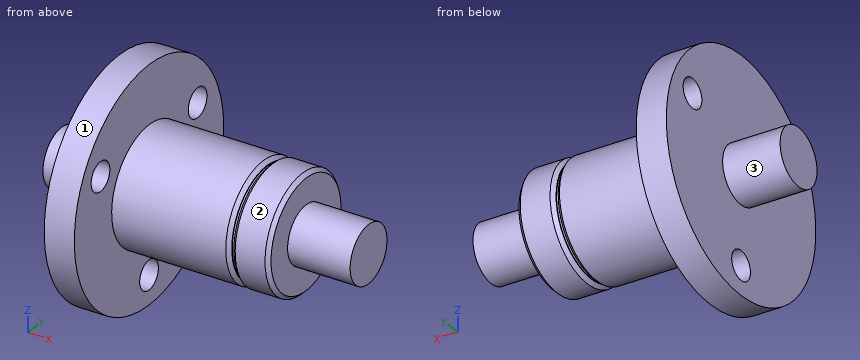
from build123d import *

# Parameters (mm, degrees)
SKETCH1_W          = 6.3
SKETCH1_H          = 3.133597909
SKETCH1_W_2        = 20.5
SKETCH1_W_3        = 6.85
SKETCH2_R          = 1.59
CUT_EXTRUDE1_DEPTH = 10
CIRPATTERN1_COUNT  = 3
CHAMFER1_SIZE      = 0.4


with BuildPart() as part:
    # Sketch1 → Revolve1 (revolve)
    with BuildSketch(Plane.XY, mode=Mode.PRIVATE) as revolve1_sk:
        with Locations((-6.45, 1.566798955)):
            Rectangle(SKETCH1_W, SKETCH1_H)
        with Locations((6.95, 1.566798955)):
            Rectangle(SKETCH1_W_2, SKETCH1_H)
        Polygon((17.2, 3.133597909), (17.2, 6.35), (13.132231879, 6.35), (13.132231879, 5.859469346), (12.9, 5.859469346), (12.9, 6.35), (0, 6.35), (0, 12.7), (-3.3, 12.7), (-3.3, 3.133597909), align=None)
        with Locations((20.625, 1.566798955)):
            Rectangle(SKETCH1_W_3, SKETCH1_H)
    revolve(revolve1_sk.sketch.rotate(Axis((-3.3, 0, 0), (1, 0, 0)), 90), axis=Axis((-3.3, 0, 0), (1, 0, 0)))

    # Sketch2 → Cut-Extrude1 (cut)
    with BuildSketch(Plane(origin=(0, 0, 0), x_dir=(0, 0, -1), z_dir=(1, 0, 0))):
        with Locations((9.525, 0)):
            Circle(SKETCH2_R)
    cut_extrude1 = extrude(amount=-CUT_EXTRUDE1_DEPTH, mode=Mode.SUBTRACT)

    # CirPattern1: Cut-Extrude1 ×3 about axis
    cirpattern1_axis = Axis((0, 0, 0), (1, 0, 0))
    for i in range(1, CIRPATTERN1_COUNT):
        add(cut_extrude1.rotate(cirpattern1_axis, i * 360 / CIRPATTERN1_COUNT), mode=Mode.SUBTRACT)

    # Chamfer1
    chamfer1_edges = [part.edges().sort_by_distance(p)[0] for p in [
        (12.9, 0, -6.35),
        (13.132231879, 0, -6.35),
        (17.2, 0, -6.35),
    ]]
    chamfer(chamfer1_edges, length=CHAMFER1_SIZE)


solid = part.part
The model under review builds one solid part; all positions refer to its coordinate system, in mm. Face numbers are marked on the shaded views. A direction names the side the tool comes from. Give positions to 0.01 mm unless a question says otherwise; leave off trailing zeros. Order: outer loops, then holes, each group sorted by start corner. A loop starts at its lowest first (then second) coordinate and runs counter-clockwise, first axis right, second up. Notation, with made-up numbers: (49.5, -17) -> (63.5, -17) arc R24 ccw to (63.5, 17) -> close; hole circle Ø5 at (-35, 56). An arc over 180 degrees is marked (long way). Write item = value, one per line. Start each with the question number.
(1) Take a section at D-D (x = 4). Write out the cut boundary in (y, z), plus the area to 3 significant figures.
(2) For L1, parallel to X at y = 2.25, z = -5.5; L2, parallel to X at y = -6.25, z = -9; L3, parallel to Y at x = -8, z = 2, list the stretches that pass through material, from the lowest coordinate up. Write a range as from..to.
(3) Take a section at C-C (y = 8). Write out the cut boundary in (x, z), plus the area to 3 significant figures.
(4) For pin 1 Ø1 at (y, z) = (-7.5, -1) entering from -X; pin 2 Ø2 at (x, z) = (2, 1.5) entering from -Y; pin 3 Ø1 at (x, y) = (12, 5.5) entering from +Z, all flat-tipped, find the tip position at first contact; note any pin that passes through.
(5) Tool access review of the marked faces 1, 2 and 3: name each direction out of +Z, -Z, +X, -X, +Y, -Y from which nothing blocks a thin tool from reaching the whole face with its end or side.
Returned:
q1.outline = circle Ø12.7 at (0, 0)
q1.area = 127 mm²
q2.L1 = -3.3..12.9, 13.13..17.2
q2.L2 = -3.3..0
q2.L3 = -2.41..2.41
q3.outline = (-3.3, -9.86) -> (0, -9.86) -> (0, 3.19) -> (-3.3, 3.19) -> close; (-3.3, 6.33) -> (0, 6.33) -> (0, 9.86) -> (-3.3, 9.86) -> close
q3.area = 54.7 mm²
q4.pin_1 = -3.3
q4.pin_2 = -6.33
q4.pin_3 = 3.91
q5.face_1 = +X, -X
q5.face_2 = +X
q5.face_3 = -X
